from build123d import *

# Parameters (mm, degrees)
ESQUISSE1_W             = 355.6
ESQUISSE1_H             = 50.8
BOSS_EXTRU_1_DEPTH      = 1
ESQUISSE2_R             = 3.96875
ENL_V_MAT_EXTRU_1_DEPTH = 1
ESQUISSE3_R             = 2.5
ENL_V_MAT_EXTRU_2_DEPTH = 2
ESQUISSE4_R             = 6.35
ENL_V_MAT_EXTRU_3_DEPTH = 2


with BuildPart() as part:
    # Esquisse1 → Boss.-Extru.1 (new body)
    with BuildSketch(Plane(origin=(0, 0, 0), x_dir=(1, 0, 0), z_dir=(0, 1, 0))):
        Rectangle(ESQUISSE1_W, ESQUISSE1_H)
    extrude(amount=BOSS_EXTRU_1_DEPTH)

    # Esquisse2 → Enlèv. mat.-Extru.1 (cut)
    with BuildSketch(Plane(origin=(0, 1, 0), x_dir=(1, 0, 0), z_dir=(0, 1, 0))):
        with Locations((-165.8, 0)):
            Circle(ESQUISSE2_R)
    extrude(amount=-ENL_V_MAT_EXTRU_1_DEPTH, mode=Mode.SUBTRACT)

    # Esquisse3 → Enlèv. mat.-Extru.2 (cut)
    with BuildSketch(Plane(origin=(0, 1, 0), x_dir=(1, 0, 0), z_dir=(0, 1, 0))):
        with Locations((-152.3, 11.55)):
            Circle(ESQUISSE3_R)
        with Locations((-129.2, 11.55)):
            Circle(ESQUISSE3_R)
        with Locations((-129.2, -11.55)):
            Circle(ESQUISSE3_R)
        with Locations((-152.3, -11.55)):
            Circle(ESQUISSE3_R)
    extrude(amount=-ENL_V_MAT_EXTRU_2_DEPTH, mode=Mode.SUBTRACT)

    # Esquisse4 → Enlèv. mat.-Extru.3 (cut)
    with BuildSketch(Plane(origin=(0, 1, 0), x_dir=(1, 0, 0), z_dir=(0, 1, 0))):
        with Locations((-76.2, 12.7)):
            Circle(ESQUISSE4_R)
        with Locations((12.7, 12.7)):
            Circle(ESQUISSE4_R)
        with Locations((12.7, -12.7)):
            Circle(ESQUISSE4_R)
        with Locations((-76.2, -12.7)):
            Circle(ESQUISSE4_R)
        with Locations((-31.75, 12.7)):
            Circle(ESQUISSE4_R)
        with Locations((57.15, 12.7)):
            Circle(ESQUISSE4_R)
        with Locations((57.15, -12.7)):
            Circle(ESQUISSE4_R)
        with Locations((-31.75, -12.7)):
            Circle(ESQUISSE4_R)
    extrude(amount=-ENL_V_MAT_EXTRU_3_DEPTH, mode=Mode.SUBTRACT)


solid = part.part
Geometry: final body of the model. Coordinates: model frame, mm. Round coordinates to 2 decimals unless told otherwise and drop trailing zeros. Loops run counter-clockwise (first coordinate to the right, second up) from the corner with the lowest first, then second, coordinate; pieces in that order, holes last. Notation, with made-up numbers: M -0.5,36 L 30.5,36 A21 ccw 30.5,57 Z; hole C -26.75,27 d9. An arc over 180 degrees is marked long. One line per question, with ' | ' between items.
(1) Material intervals for line 1 along Z through (x, y) = (57.15, 0.25); line 2 along Z through (x, y) = (-129.5, 0.9); line 3 along Z through (x, y) = (-165.8, 0.3), sorted ascending. Write a range as from..to.
Check result:
line 1: z = -25.4..-19.05, -6.35..6.35, 19.05..25.4 | line 2: z = -25.4..-14.03, -9.07..9.07, 14.03..25.4 | line 3: z = -25.4..-3.97, 3.97..25.4
(2) Pull-direction query (Z, two-part tool) for faces 1 (the cylindrical face through (-82.544, 0.507, 12.421)), 2 (the flat face through (-2, 0, 0)); classes: +Z half, -Z half, draft (parallel to the pull), parting line (faces both ways), or undercut.
Check result:
face 1: undercut | face 2: draft
(3) Cut plane A-A on x = 12.7. Return the cut outline in (y, z).
Check result:
outline: M 0,-25.4 L 1,-25.4 L 1,-19.05 L 0,-19.05 Z; M 0,-6.35 L 1,-6.35 L 1,6.35 L 0,6.35 Z; M 0,19.05 L 1,19.05 L 1,25.4 L 0,25.4 Z
(4) Cut plane B-B on y = 0.25. Give the number of separate pieces and of enclosed holes in the cut face, plus the area to 3 significant figures.
Check result:
separate pieces: 1 | enclosed holes: 13 | area: 16,900 mm2
